For this review, take the finished solid that the model builds, in its own axes (mm). A direction names the side the tool comes from. Coordinates: 2 decimals unless noted, no trailing zeros. Loops run counter-clockwise (first coordinate to the right, second up) from the corner with the lowest first, then second, coordinate; pieces in that order, holes last. Notation, with made-up numbers: (10, 29) -> (21, 29) arc R5 cw to (21, 38) -> close; hole circle Ø6 at (72.5, -39.75). An arc over 180 degrees is marked (long way). Use a Markdown table: item, result.
from build123d import *

# Parameters (mm, degrees)
SKETCH1_W           = 90
SKETCH1_H           = 120
SKETCH1_R           = 24.5
SKETCH1_W_2         = 10
SKETCH1_H_2         = 40
SKETCH1_W_3         = 40
SKETCH1_H_3         = 10
BOSS_EXTRUDE1_DEPTH = 5


with BuildPart() as part:
    # Sketch1 → Boss-Extrude1 (new body)
    # profile 1 of 5: a face of its own
    with BuildSketch(Plane(origin=(0, 0, 0), x_dir=(1, 0, 0), z_dir=(0, 1, 0))):
        with Locations((45, 60)):
            Rectangle(SKETCH1_W, SKETCH1_H)
        with Locations(Location((36.72, 31.48, 0), (0, 0, 270))):
            Circle(SKETCH1_R, mode=Mode.SUBTRACT)
    # profile 2 of 5: a face of its own
    with BuildSketch(Plane(origin=(0, 0, 0), x_dir=(1, 0, 0), z_dir=(0, 1, 0))):
        with Locations((-5, 60)):
            Rectangle(SKETCH1_W_2, SKETCH1_H_2)
    # profile 3 of 5: a face of its own
    with BuildSketch(Plane(origin=(0, 0, 0), x_dir=(1, 0, 0), z_dir=(0, 1, 0))):
        with Locations((45, 125)):
            Rectangle(SKETCH1_W_3, SKETCH1_H_3)
    # profile 4 of 5: a face of its own
    with BuildSketch(Plane(origin=(0, 0, 0), x_dir=(1, 0, 0), z_dir=(0, 1, 0))):
        with Locations((95, 60)):
            Rectangle(SKETCH1_W_2, SKETCH1_H_2)
    # profile 5 of 5: a face of its own
    with BuildSketch(Plane(origin=(0, 0, 0), x_dir=(1, 0, 0), z_dir=(0, 1, 0))):
        with Locations((45, -5)):
            Rectangle(SKETCH1_W_3, SKETCH1_H_3)
    extrude(amount=BOSS_EXTRUDE1_DEPTH)


solid = part.part
(1) Take a section at C-C on y = 3.15. Write out the cut boundary in (x, z), plus the area to 3 significant figures.
Found:
| item | result |
|---|---|
| outline | (-10, -80) -> (0, -80) -> (0, -120) -> (25, -120) -> (25, -130) -> (65, -130) -> (65, -120) -> (90, -120) -> (90, -80) -> (100, -80) -> (100, -40) -> (90, -40) -> (90, 0) -> (65, 0) -> (65, 10) -> (25, 10) -> (25, 0) -> (0, 0) -> (0, -40) -> (-10, -40) -> close; hole circle Ø49 at (36.72, -31.48) |
| area | 10,500 mm^2 |
(2) Take a section at A-A on z = -31.48. Write out the cut boundary in (x, y), plus the area to 3 significant figures.
Found:
| item | result |
|---|---|
| outline | (0, 0) -> (12.22, 0) -> (12.22, 5) -> (0, 5) -> close; (61.22, 0) -> (90, 0) -> (90, 5) -> (61.22, 5) -> close |
| area | 205 mm^2 |
(3) For faces 4 (the face through (12, 2, 0)), 5 (the face through (25, 2, -125)), 6 (the face through (77, 2, -120)), 7 (the face through (77, 2, 0)), list the 3-axis set-ups (+Z, -Z, +X, -X, +Y, -Y) from which the entire face can be reached by the end or side of a thin tool; tool diameter is ignored.
Found:
| item | result |
|---|---|
| face 4 | +Z, -X, +Y, -Y |
| face 5 | -Z, -X, +Y, -Y |
| face 6 | -Z, +X, +Y, -Y |
| face 7 | +Z, +X, +Y, -Y |
(4) Mouldability with a two-part tool opening along Z and no side actions: class faces 1 (the face through (65, 2, -125)), 2 (the face through (57.38, 2.46, -18.31)), 3 (the face through (95, 2, -40)) as pulls with the +Z half, pulls with the -Z half, needs draft (parallel to the pull), parting line crosses it, or undercut.
Found:
| item | result |
|---|---|
| face 1 | needs draft |
| face 2 | undercut |
| face 3 | pulls with the +Z half |
(5) For line 1 along X through (y, z) = (3.2, -31.48); line 2 along Z through (x, y) = (38, 4.7); line 3 along X through (y, z) = (3, -104), list the stretches that pass through material, from the lowest coordinate up.
Found:
| item | result |
|---|---|
| line 1 | x = 0 to 12.22, 61.22 to 90 |
| line 2 | z = -130 to -55.95, -7.01 to 10 |
| line 3 | x = 0 to 90 |
(6) Take a section at D-D on z = -94. Write out the cut boundary in (x, y).
Found:
| item | result |
|---|---|
| outline | (0, 0) -> (90, 0) -> (90, 5) -> (0, 5) -> close |
(7) For pin 1 Ø1 at (y, z) = (1.5, -16) entering from -X; pin 2 Ø1.5 at (x, y) = (72.5, 2.5) entering from +Z; pin 3 Ø2.5 at (y, z) = (2.5, -127) entering from +X, all flat-tipped, find the tip position at first contact; note any pin that passes through.
Found:
| item | result |
|---|---|
| pin 1 | stops at x = 0 |
| pin 2 | stops at z = 0 |
| pin 3 | stops at x = 65 |
(8) Take a section at B-B on x = 36.72. Write out the cut boundary in (y, z).
Found:
| item | result |
|---|---|
| outline | (0, -130) -> (5, -130) -> (5, -55.98) -> (0, -55.98) -> close; (0, -6.98) -> (5, -6.98) -> (5, 10) -> (0, 10) -> close |
